Model file for the job. Use its own axes, mm. A direction names the side the tool comes from. Coordinates: 2 decimals unless noted, no trailing zeros.
Q1. Band-saw the part on A-A, the plane z = 44.5. State how many separate pieces and enclosed holes the cut face has, plus the area to 3 significant figures.
Q2. Pull direction X, two halves, no side cores. Call faces 3 (the flat face through (-12.7, 0, 5)), 4 (the flat face through (-10.49, 0, 5)), 5 (the flat face through (-3, 0, 355.6)): released by +X, released by -X, zero draft, split by the parting line, or undercut.
Q3. Which spindle directions (+Z, -Z, +X, -X, +Y, -Y) get a long thin tool onto all of the face, cutting with end or side? Do faces 1 (the flat face through (-3, 0, -355.6)), 2 (the flat face through (0, -10.49, 5)). Say none if no direction does.
Q4. Drill centre lines: probe 1 along Y at (x, z) = (0, -16.5); probe 2 along Y at (x, z) = (-9, -10); probe 3 along Y at (x, z) = (-5.5, 135.5). Where is each one in solid material? Low to high.
Q5. Pin check, flat tips, straight feed: P1, Ø1, axis at x = 2.5, z = -131, coming from the +Y side; P2, Ø1.1, axis at y = 0, z = 99.5, coming from the +X side; P3, Ø4, axis at x = -2, z = -177.5, coming from the +Y side. Stop position of each tip, or through.
from build123d import *

# Parameters (mm, degrees)
SKETCH3_R      = 2.6035
EXTRUDE1_DEPTH = 355.6


with BuildPart() as part:
    # Sketch3 → Extrude1 (new, symmetric)
    with BuildSketch(Plane.XY):
        with BuildLine():
            Line((-1.115277175, 4.5085), (1.115277175, 4.5085))
            ThreePointArc((1.115277175, 4.5085), (2.806584872, 4.844922018), (4.240406305, 5.80297087))
            Line((4.240406305, 5.80297087), (7.119225992, 8.681790557))
            ThreePointArc((7.119225992, 8.681790557), (7.348862413, 9.836250802), (6.370158275, 10.4902))
            Line((6.370158275, 10.4902), (4.3434, 10.4902))
            ThreePointArc((4.3434, 10.4902), (3.2385, 11.5951), (4.3434, 12.7))
            Line((4.3434, 12.7), (5.738786846, 12.7))
            ThreePointArc((5.738786846, 12.7), (6.054472561, 12.384314286), (6.370158275, 12.7))
            Line((6.370158275, 12.7), (9.858828571, 12.7))
            ThreePointArc((9.858828571, 12.7), (10.174514286, 12.384314286), (10.4902, 12.7))
            ThreePointArc((10.4902, 12.7), (12.052764565, 12.052764565), (12.7, 10.4902))
            ThreePointArc((12.7, 10.4902), (12.384314286, 10.174514286), (12.7, 9.858828571))
            Line((12.7, 9.858828571), (12.7, 6.370158275))
            ThreePointArc((12.7, 6.370158275), (12.384314286, 6.054472561), (12.7, 5.738786846))
            Line((12.7, 5.738786846), (12.7, 4.3434))
            ThreePointArc((12.7, 4.3434), (11.5951, 3.2385), (10.4902, 4.3434))
            Line((10.4902, 4.3434), (10.4902, 6.370158275))
            ThreePointArc((10.4902, 6.370158275), (9.836250802, 7.348862413), (8.681790557, 7.119225992))
            Line((8.681790557, 7.119225992), (5.80297087, 4.240406305))
            ThreePointArc((5.80297087, 4.240406305), (4.844922018, 2.806584872), (4.5085, 1.115277175))
            Line((4.5085, 1.115277175), (4.5085, -1.115277175))
            ThreePointArc((4.5085, -1.115277175), (4.844922018, -2.806584872), (5.80297087, -4.240406305))
            Line((5.80297087, -4.240406305), (8.681790557, -7.119225992))
            ThreePointArc((8.681790557, -7.119225992), (9.836250802, -7.348862413), (10.4902, -6.370158275))
            Line((10.4902, -6.370158275), (10.4902, -4.3434))
            ThreePointArc((10.4902, -4.3434), (11.5951, -3.2385), (12.7, -4.3434))
            Line((12.7, -4.3434), (12.7, -5.738786846))
            ThreePointArc((12.7, -5.738786846), (12.384314286, -6.054472561), (12.7, -6.370158275))
            Line((12.7, -6.370158275), (12.7, -9.858828571))
            ThreePointArc((12.7, -9.858828571), (12.384314286, -10.174514286), (12.7, -10.4902))
            ThreePointArc((12.7, -10.4902), (12.052764565, -12.052764565), (10.4902, -12.7))
            ThreePointArc((10.4902, -12.7), (10.174514286, -12.384314286), (9.858828571, -12.7))
            Line((9.858828571, -12.7), (6.370158275, -12.7))
            ThreePointArc((6.370158275, -12.7), (6.054472561, -12.384314286), (5.738786846, -12.7))
            Line((5.738786846, -12.7), (4.3434, -12.7))
            Line((4.3434, -12.7), (-5.738786846, -12.7))
            ThreePointArc((-5.738786846, -12.7), (-6.054472561, -12.384314286), (-6.370158275, -12.7))
            Line((-6.370158275, -12.7), (-9.858828571, -12.7))
            ThreePointArc((-9.858828571, -12.7), (-10.174514286, -12.384314286), (-10.4902, -12.7))
            ThreePointArc((-10.4902, -12.7), (-12.052764565, -12.052764565), (-12.7, -10.4902))
            ThreePointArc((-12.7, -10.4902), (-12.384314286, -10.174514286), (-12.7, -9.858828571))
            Line((-12.7, -9.858828571), (-12.7, -6.370158275))
            ThreePointArc((-12.7, -6.370158275), (-12.384314286, -6.054472561), (-12.7, -5.738786846))
            Line((-12.7, -5.738786846), (-12.7, 0))
            Line((-12.7, 0), (-12.7, 5.738786846))
            ThreePointArc((-12.7, 5.738786846), (-12.384314286, 6.054472561), (-12.7, 6.370158275))
            Line((-12.7, 6.370158275), (-12.7, 9.858828571))
            ThreePointArc((-12.7, 9.858828571), (-12.384314286, 10.174514286), (-12.7, 10.4902))
            ThreePointArc((-12.7, 10.4902), (-12.052764565, 12.052764565), (-10.4902, 12.7))
            ThreePointArc((-10.4902, 12.7), (-10.174514286, 12.384314286), (-9.858828571, 12.7))
            Line((-9.858828571, 12.7), (-6.370158275, 12.7))
            ThreePointArc((-6.370158275, 12.7), (-6.054472561, 12.384314286), (-5.738786846, 12.7))
            Line((-5.738786846, 12.7), (-4.3434, 12.7))
            ThreePointArc((-4.3434, 12.7), (-3.2385, 11.5951), (-4.3434, 10.4902))
            Line((-4.3434, 10.4902), (-6.370158275, 10.4902))
            ThreePointArc((-6.370158275, 10.4902), (-7.348862413, 9.836250802), (-7.119225992, 8.681790557))
            Line((-7.119225992, 8.681790557), (-4.240406305, 5.80297087))
            ThreePointArc((-4.240406305, 5.80297087), (-2.806584872, 4.844922018), (-1.115277175, 4.5085))
        make_face()
        Circle(SKETCH3_R, mode=Mode.SUBTRACT)
        with BuildLine():
            Line((-4.5085, -1.115277175), (-4.5085, 1.115277175))
            ThreePointArc((-4.5085, 1.115277175), (-4.844922018, 2.806584872), (-5.80297087, 4.240406305))
            Line((-5.80297087, 4.240406305), (-8.681790557, 7.119225992))
            ThreePointArc((-8.681790557, 7.119225992), (-9.836250802, 7.348862413), (-10.4902, 6.370158275))
            Line((-10.4902, 6.370158275), (-10.4902, 0))
            Line((-10.4902, 0), (-10.4902, -6.370158275))
            ThreePointArc((-10.4902, -6.370158275), (-9.836250802, -7.348862413), (-8.681790557, -7.119225992))
            Line((-8.681790557, -7.119225992), (-5.80297087, -4.240406305))
            ThreePointArc((-5.80297087, -4.240406305), (-4.844922018, -2.806584872), (-4.5085, -1.115277175))
        make_face(mode=Mode.SUBTRACT)
        with BuildLine():
            Line((4.240406305, -5.80297087), (7.119225992, -8.681790557))
            ThreePointArc((7.119225992, -8.681790557), (7.348862413, -9.836250802), (6.370158275, -10.4902))
            Line((6.370158275, -10.4902), (4.3434, -10.4902))
            Line((4.3434, -10.4902), (-6.370158275, -10.4902))
            ThreePointArc((-6.370158275, -10.4902), (-7.348862413, -9.836250802), (-7.119225992, -8.681790557))
            Line((-7.119225992, -8.681790557), (-4.240406305, -5.80297087))
            ThreePointArc((-4.240406305, -5.80297087), (-2.806584872, -4.844922018), (-1.115277175, -4.5085))
            Line((-1.115277175, -4.5085), (1.115277175, -4.5085))
            ThreePointArc((1.115277175, -4.5085), (2.806584872, -4.844922018), (4.240406305, -5.80297087))
        make_face(mode=Mode.SUBTRACT)
    extrude(amount=EXTRUDE1_DEPTH, both=True)


solid = part.part
Answer sheet:
1. separate pieces: 1
1. enclosed holes: 3
1. area: 317 mm2
2. face 3: released by -X
2. face 4: undercut
2. face 5: zero draft
3. face 1: -Z, +X, -X, +Y, -Y
3. face 2: +Z, -Z
4. probe 1: y = -12.7 to -10.49, -4.51 to -2.6, 2.6 to 4.51
4. probe 2: y = -12.7 to -7.34, 7.34 to 12.7
4. probe 3: y = -12.7 to -10.49, -7.06 to -3.9, 3.9 to 7.06, 10.49 to 12.7
5. P1: stops at y = 4.93
5. P2: stops at x = 4.51
5. P3: stops at y = 12.65
